Drawing for the job (mm, zero at the part's lowest x, y, z). A direction names the side the tool comes from. Give positions to 0.01 mm unless a question says otherwise; leave off trailing zeros. Loops run counter-clockwise (first coordinate to the right, second up) from the corner with the lowest first, then second, coordinate; pieces in that order, holes last. Notation, with made-up numbers: (-24.5, 72) - (-15.5, 72) arc R17 ccw to (-15.5, 101) - close; hole circle Ø8 at (-38.5, 74). An arc over 180 degrees is marked (long way). Return JSON: item names as keys, results as strings. Group by question number.
1) Slice it at B-B (z = 77). Count the separate pieces of the cut face and the enclosed holes in it, and give its area (3 significant figures).
2) Drop a flat-ended pin along its axis: pin 1 (3 mm diameter, centred on x = 609.5, y = 628, fed in from +Z). Give the stop position or say it passes through.
3) Drill centre lines: probe 1 along Y at (x, z) = (466.5, 69.5); probe 2 along Z at (x, y) = (267.5, 631). Where is each one in solid material? Low to high. Write a range as from..to.
4) Slice it at A-A (y = 721.5). List the corners of the cut face in (x, z), and give its area (3 significant figures).
5) Mould opens along X. For the marked faces 3 and 4 say: released by +X, released by -X, zero draft, split by the parting line, or undercut.
6) 3-axis set-ups, long thin cutter, end or side, ignore diameter. For the marked faces 1 and 2: which of +Z, -Z, +X, -X, +Y, -Y reach the whole face in a straight line?
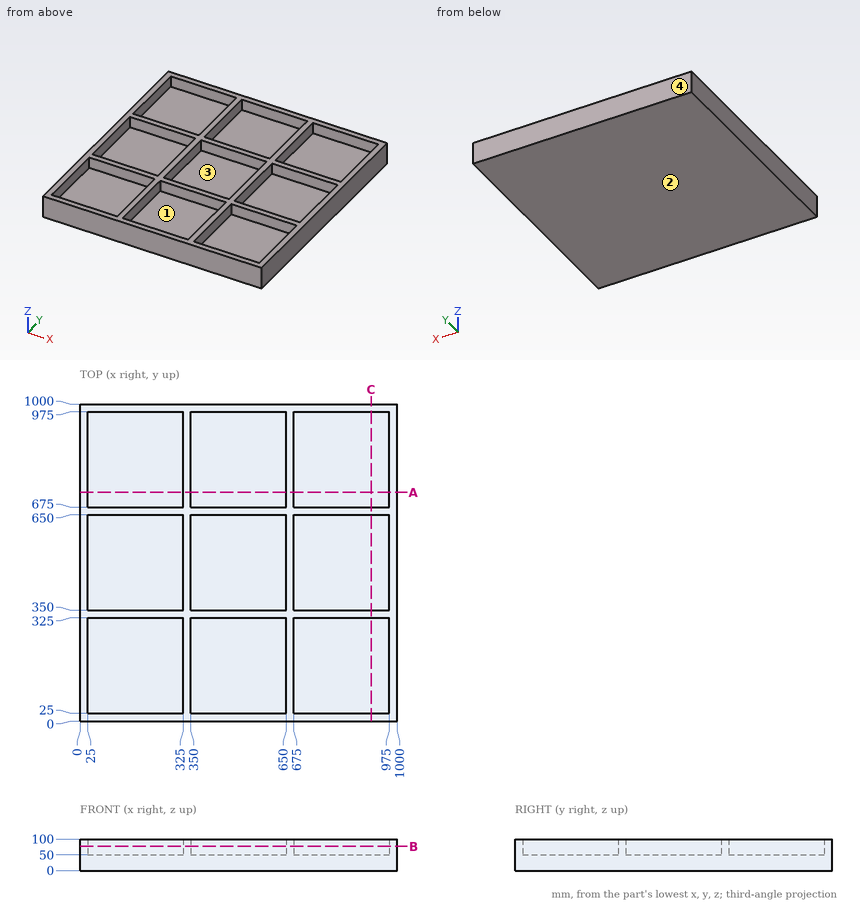
Results:
{
 "1": {"separate pieces": "1", "enclosed holes": "9", "area": "190,000 mm2"},
 "2": {"pin 1": "z = 50"},
 "3": {"probe 1": "0..25, 325..350, 650..675, 975..1000", "probe 2": "0..50"},
 "4": {"outline": "(0, 0) - (1000, 0) - (1000, 100) - (975, 100) - (975, 50) - (675, 50) - (675, 100) - (650, 100) - (650, 50) - (350, 50) - (350, 100) - (325, 100) - (325, 50) - (25, 50) - (25, 100) - (0, 100) - close", "area": "55,000 mm2"},
 "5": {"face 3": "undercut", "face 4": "zero draft"},
 "6": {"face 1": "+Z", "face 2": "-Z, +X, -X, +Y, -Y"}
}
